```python
from build123d import *

# Parameters (mm, degrees)
BOSS_EXTRUDE3_DEPTH = 10
BOSS_EXTRUDE4_DEPTH = 1
CUT_EXTRUDE1_START  = -9
SKETCH3_R           = 4
SKETCH3_R_2         = 1.5
CUT_EXTRUDE1_DEPTH  = 9
SKETCH4_W           = 2.809732667
SKETCH4_H           = 2
CUT_EXTRUDE2_DEPTH  = 8
SKETCH5_W           = 2.809732667
SKETCH5_H           = 2
BOSS_EXTRUDE5_DEPTH = 1
BOSS_EXTRUDE6_START = -8
BOSS_EXTRUDE6_DEPTH = 8
FILLET3_R           = 1


with BuildPart() as part:
    # Sketch1 → Boss-Extrude3 (new body)
    with BuildSketch(Plane(origin=(0, 0, 0), x_dir=(0, 0, -1), z_dir=(1, 0, 0))):
        with BuildLine():
            Line((7.708712153, -1), (4.898979486, -1))
            ThreePointArc((4.898979486, -1), (-5, 0), (4.898979486, 1))
            Line((4.898979486, 1), (7.708712153, 1))
            ThreePointArc((7.708712153, 1), (12.5, 0), (7.708712153, -1))
        make_face()
        with BuildLine():
            ThreePointArc((8.881966011, -1), (11.5, 0), (8.881966011, 1))
            Line((8.881966011, 1), (8.881966011, 0.5))
            Line((8.881966011, 0.5), (3.872983346, 0.5))
            Line((3.872983346, 0.5), (3.872983346, 1))
            ThreePointArc((3.872983346, 1), (-4, 0), (3.872983346, -1))
            Line((3.872983346, -1), (3.872983346, -0.5))
            Line((3.872983346, -0.5), (8.881966011, -0.5))
            Line((8.881966011, -0.5), (8.881966011, -1))
        make_face(mode=Mode.SUBTRACT)
    extrude(amount=BOSS_EXTRUDE3_DEPTH)

    # Sketch2 → Boss-Extrude4 (add)
    with BuildSketch(Plane.ZY):
        with BuildLine():
            Line((-8.585786438, 0.5), (-3.968626967, 0.5))
            ThreePointArc((-3.968626967, 0.5), (4, 0), (-3.968626967, -0.5))
            Line((-3.968626967, -0.5), (-8.585786438, -0.5))
            ThreePointArc((-8.585786438, -0.5), (-11.5, 0), (-8.585786438, 0.5))
        make_face()
    extrude(amount=-BOSS_EXTRUDE4_DEPTH)

    # Sketch3 → Cut-Extrude1 (cut)
    with BuildSketch(Plane(origin=(10, 0, 0), x_dir=(0, 0, -1), z_dir=(1, 0, 0)).offset(CUT_EXTRUDE1_START)):
        Circle(SKETCH3_R)
        with Locations((10, 0)):
            Circle(SKETCH3_R_2)
    extrude(amount=CUT_EXTRUDE1_DEPTH, mode=Mode.SUBTRACT)

    # Sketch4 → Cut-Extrude2 (cut)
    with BuildSketch(Plane(origin=(10, 0, 0), x_dir=(0, 0, -1), z_dir=(1, 0, 0))):
        with Locations((6.30384582, 0)):
            Rectangle(SKETCH4_W, SKETCH4_H)
    extrude(amount=-CUT_EXTRUDE2_DEPTH, mode=Mode.SUBTRACT)

    # Sketch5 → Boss-Extrude5 (add)
    with BuildSketch(Plane(origin=(2, 0, 0), x_dir=(0, 0, -1), z_dir=(1, 0, 0))):
        with Locations((6.30384582, 0)):
            Rectangle(SKETCH5_W, SKETCH5_H)
    extrude(amount=BOSS_EXTRUDE5_DEPTH)

    # Sketch6 → Boss-Extrude6 (add)
    with BuildSketch(Plane(origin=(10, 0, 0), x_dir=(0, 0, -1), z_dir=(1, 0, 0)).offset(BOSS_EXTRUDE6_START)):
        with BuildLine():
            Line((3.968626967, 0.5), (4.969531559, 0.5))
            ThreePointArc((4.969531559, 0.5), (4.994621499, 0), (4.969531559, -0.5))
            Line((4.969531559, -0.5), (3.968626967, -0.5))
            ThreePointArc((3.968626967, -0.5), (4, 0), (3.968626967, 0.5))
        make_face()
        with BuildLine():
            Line((8.585786438, 0.5), (7.550510257, 0.5))
            ThreePointArc((7.550510257, 0.5), (7.5, 0), (7.550510257, -0.5))
            Line((7.550510257, -0.5), (8.585786438, -0.5))
            ThreePointArc((8.585786438, -0.5), (8.5, 0), (8.585786438, 0.5))
        make_face()
    extrude(amount=BOSS_EXTRUDE6_DEPTH)

    # Fillet3
    # the kernel refuses this fillet: 1 mm, written as the material it takes off along each edge
    with BuildSketch(Plane(origin=(3, 0.5, -4.969531559), x_dir=(0, -0.9982310173351231, -0.059454487047532374), z_dir=(1, 0, 0))) as fillet3_piece_1:
        with BuildLine():
            CenterArc((0.366534345, -0.999168363), FILLET3_R, 87.663129738, 24.097452775)
            Line((-0.004194637, -0.070427268), (0, 0))
            ThreePointArc((0, 0), (0.203654559, 0.004153711), (0.407309118, 0))
        make_face()
    extrude(amount=8.018272795, mode=Mode.SUBTRACT)
    with BuildSketch(Plane(origin=(3, -0.5, -4.969531559), x_dir=(0, 0, 1), z_dir=(1, 0, 0))) as fillet3_piece_2:
        with BuildLine():
            CenterArc((0.97560874, -0.425290994), FILLET3_R, 154.830916209, 24.097452775)
            ThreePointArc((-0.024216355, -0.406588595), (-0.016254541, -0.203047341), (0, 0))
            Line((0, 0), (0.070552073, 0))
        make_face()
    extrude(amount=8.018272795, mode=Mode.SUBTRACT)
    with BuildSketch(Plane(origin=(3, -0.5, -7.550510257), x_dir=(0, 8.127970304186451e-12, -1.0), z_dir=(1, 0, 0))) as fillet3_piece_3:
        with BuildLine():
            CenterArc((0.953276133, 0.606512125), FILLET3_R, 175.928109784, 41.40962211)
            ThreePointArc((-0.044199608, 0.677520208), (-0.045207292, 0.337252633), (0, 0))
            Line((0, 0), (0.158201895, 0))
        make_face()
    extrude(amount=8.697401022, mode=Mode.SUBTRACT)
    with BuildSketch(Plane(origin=(3, 0.5, -7.550510257), x_dir=(0, -0.9978788138478943, 0.06509894679270496), z_dir=(1, 0, 0))) as fillet3_piece_4:
        with BuildLine():
            CenterArc((0.543168327, 0.990737357), FILLET3_R, 236.394802514, 41.40962211)
            Line((-0.010298777, 0.15786632), (0, 0))
            ThreePointArc((0, 0), (0.339480204, -0.023156608), (0.678960409, 0))
        make_face()
    extrude(amount=8.697401022, mode=Mode.SUBTRACT)


solid = part.part
```
For this review, take the finished solid that the model builds, in its own axes (mm). A direction names the side the tool comes from. Round coordinates to 2 decimals unless told otherwise and drop trailing zeros. Write each loop counter-clockwise with the first axis right and the second up, starting at its lowest first coordinate (ties: lowest second). Pieces come first, ordered by that corner, then holes.
1) Machinability: for faces 3 (the face through (1, 1, -6)), 4 (the face through (2, 0, -6)), 5 (the face through (1, -1, -6)), 6 (the face through (4.9, 0.1, -12.5)), which of the approach directions +Z, -Z, +X, -X, +Y, -Y give a long, thin tool a straight path to every point of the face, cutting with its end or side? Answer none if there is none.
Answer below:
face 3: +X, -X, +Y
face 4: none
face 5: +X, -X, -Y
face 6: +X, -X
2) Insertion check: pin 1 Ø6 at (x, y) = (3, -3.5) entering from -Z; pin 2 Ø6 at (x, z) = (9, -5) entering from -Y; pin 3 Ø0.5 at (x, z) = (1.5, -6) entering from -Y. Each pin has a flat end and moves straight along its axis. Give the tip position at first contact, or say it passes through.
Answer below:
pin 1: stops at z = -12.45
pin 2: stops at y = -4.58
pin 3: stops at y = -1
3) Mouldability with a two-part tool opening along Z and no side actions: class faces 1 (the face through (1.5, 0.5, -6.3)), 2 (the face through (0, 0, -2)) as +Z half, -Z half, draft (parallel to the pull), parting line (faces both ways), or undercut.
Answer below:
face 1: undercut
face 2: draft
4) Take a section at B-B on y = 2. Give the boundary of the cut face in (x, z).
Answer below:
outline: (0, -11.5) - (10, -11.5) - (10, -8.5) - (0, -8.5) - close; (0, -4.58) - (10, -4.58) - (10, -3.46) - (1, -3.46) - (1, 3.46) - (10, 3.46) - (10, 4.58) - (0, 4.58) - close
5) Take a section at D-D on x = 2.5. Give the boundary of the cut face in (y, z), then the cut area to 3 significant figures.
Answer below:
outline: (-1, -7.71) arc R2.5 ccw (long way) to (1, -7.71) - (1, -4.9) arc R5 ccw (long way) to (-1, -4.9) - close; hole circle Ø8 at (0, 0); hole circle Ø3 at (0, -10)
area: 46.0 mm2
6) Take a section at A-A on x = 9.5. Give the boundary of the cut face in (y, z).
Answer below:
outline: (-1, -7.71) arc R2.5 ccw (long way) to (1, -7.71) - (0.5, -7.71) arc R1 ccw to (0, -7.51) arc R1 ccw to (-0.5, -7.71) - close; (-1, -4.9) - (-0.5, -4.9) arc R1 ccw to (-0.09, -4.99) arc R4.99 ccw to (0.09, -4.99) arc R1 ccw to (0.5, -4.9) - (1, -4.9) arc R5 ccw (long way) to start; hole circle Ø8 at (0, 0); hole circle Ø3 at (0, -10)
7) Take a section at C-C on z = -10. Give the boundary of the cut face in (x, y).
Answer below:
outline: (0, -2.5) - (10, -2.5) - (10, -1.5) - (1, -1.5) - (1, 1.5) - (10, 1.5) - (10, 2.5) - (0, 2.5) - close
8) For line 1 along Y through (x, z) = (6.25, -10); line 2 along Y through (x, z) = (1.5, -6); line 3 along X through (y, z) = (-1.25, -2.25), list the stretches that pass through material, from the lowest coordinate up.
Answer below:
line 1: y = -2.5 to -1.5, 1.5 to 2.5
line 2: y = -1 to -0.5, 0.5 to 1
line 3: x = 0 to 1
